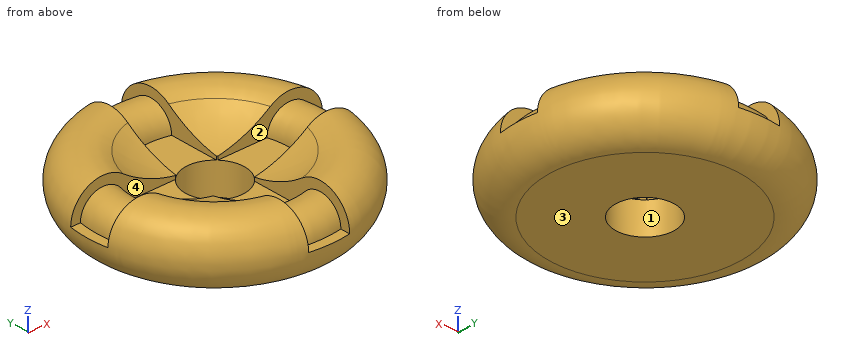
from build123d import *

# Parameters (mm, degrees)
F3_W     = 6.428574
F3_H     = 17.960521
F3_W_2   = 17.799999
F3_H_2   = 6.428573
F3_W_3   = 18.051646
F3_H_3   = 17.891126
F4_DEPTH = 5
F5_R     = 3.5
F7_R     = 4.602203
F8_DEPTH = 25


with BuildPart() as f1:
    # F0 (on Front) → F1 (revolve)
    with BuildSketch(Plane.XZ):
        with BuildLine():
            ThreePointArc((0, 5), (-6.324555, 6.026334), (-12, 9))
            ThreePointArc((-12, 9), (-19.743416, 6.581139), (-15, 0))
            Line((-15, 0), (0, 0))
            Line((0, 0), (0, 5))
        make_face()
    revolve(axis=Axis((0, 0, 2.5), (0, 0, 1)))

    # F3 (on offset) → F4 (cut)
    with BuildSketch(Plane.XY.offset(10)):
        with Locations((0, 12.159849)):
            Rectangle(F3_W, F3_H)
        with Locations((12.114286, -0.034697)):
            Rectangle(F3_W_2, F3_H_2)
        with Locations((-12.24011, -0.034697)):
            Rectangle(F3_W_3, F3_H_2)
        with Locations((0, -12.194547)):
            Rectangle(F3_W, F3_H_3)
    extrude(amount=-F4_DEPTH, mode=Mode.SUBTRACT)

    # F5 (on Front) → F6 (revolve)
    with BuildSketch(Plane.XZ):
        with Locations((-15, 5)):
            Circle(F5_R)
    revolve(axis=Axis((0, 0, 2.5), (0, 0, 1)))

    # F7 (on offset) → F8 (cut)
    with BuildSketch(Plane.XY.offset(10)):
        Circle(F7_R)
    extrude(amount=-F8_DEPTH, mode=Mode.SUBTRACT)


solid = f1.part
Design review of the part built by this model. Coordinates are the model's own, in mm. Face numbers are marked on the shaded views. A direction names the side the tool comes from. Give positions to 0.01 mm unless a question says otherwise; leave off trailing zeros. Loops run counter-clockwise (first coordinate to the right, second up) from the corner with the lowest first, then second, coordinate; pieces in that order, holes last. Notation, with made-up numbers: (48, -19.75) - (75, -19.75) arc R33 ccw to (75, 17.25) - close; hole circle Ø1 at (53, -23.5). An arc over 180 degrees is marked (long way). Use CSV: the item, a comma, the result in double quotes. Start each with the question number.
1. Draft analysis for pull direction Y (two halves, no side actions). For the marked faces 3 and 4, state which applies: released by +Y, released by -Y, zero draft, split by the parting line, or undercut.
2. Add section A-A (y = 0). State the section outline as (x, z) points.
3. Wall thickness on L1, parallel to X at y = 0, z = 3.75; L2, parallel to X at y = 0, z = 1.2; L3, parallel to Y at x = -6, z = 8: over which ranges is each line inside the solid? List them lowest first.
4. Machinability: for the marked faces 1 and 2, which of the approach directions +Z, -Z, +X, -X, +Y, -Y give a long, thin tool a straight path to every point of the face, cutting with its end or side? Answer none if there is none.
5. Insertion check: P1, Ø7, axis at x = -7.5, y = 0, coming from the +Z side; P2, Ø2.5, axis at y = 9, z = 8, coming from the -X side (3 decimals); P3, Ø2, axis at y = 11.5, z = 8, coming from the +X side; P4, Ø7.5, axis at x = 0, y = 0, coming from the +Z side. Each pin has a flat end and moves straight along its axis. Give the tip position at first contact, or say it passes through.
6. Add section D-D (z = 4). State the section outline as (x, y) points.
7. Add section C-C (z = 1.5). State the section outline as (x, y) points.
Results found:
1,face 3,"zero draft"
1,face 4,"undercut"
2,outline,"(-20, 5) arc R5 ccw to (-15, 0) - (-4.6, 0) - (-4.6, 5) - (-11.5, 5) arc R3.5 ccw to (-18.5, 5) - close; (4.6, 0) - (15, 0) arc R5 ccw to (20, 5) - (18.5, 5) arc R3.5 ccw to (11.5, 5) - (4.6, 5) - close"
3,L1,"x = -19.84 to -4.6, 4.6 to 19.84"
3,L2,"x = -18.25 to -4.6, 4.6 to 18.25"
3,L3,"y = -18.03 to -8.66, 8.66 to 18.03"
4,face 1,"+Z, -Z"
4,face 2,"+Z"
5,P1,"stops at z = 7.41"
5,P2,"stops at x = -17.765"
5,P3,"stops at x = 16.17"
5,P4,"passes through"
6,outline,"circle Ø39.8 at (0, 0); hole circle Ø9.2 at (0, 0)"
7,outline,"circle Ø37.14 at (0, 0); hole circle Ø9.2 at (0, 0)"
